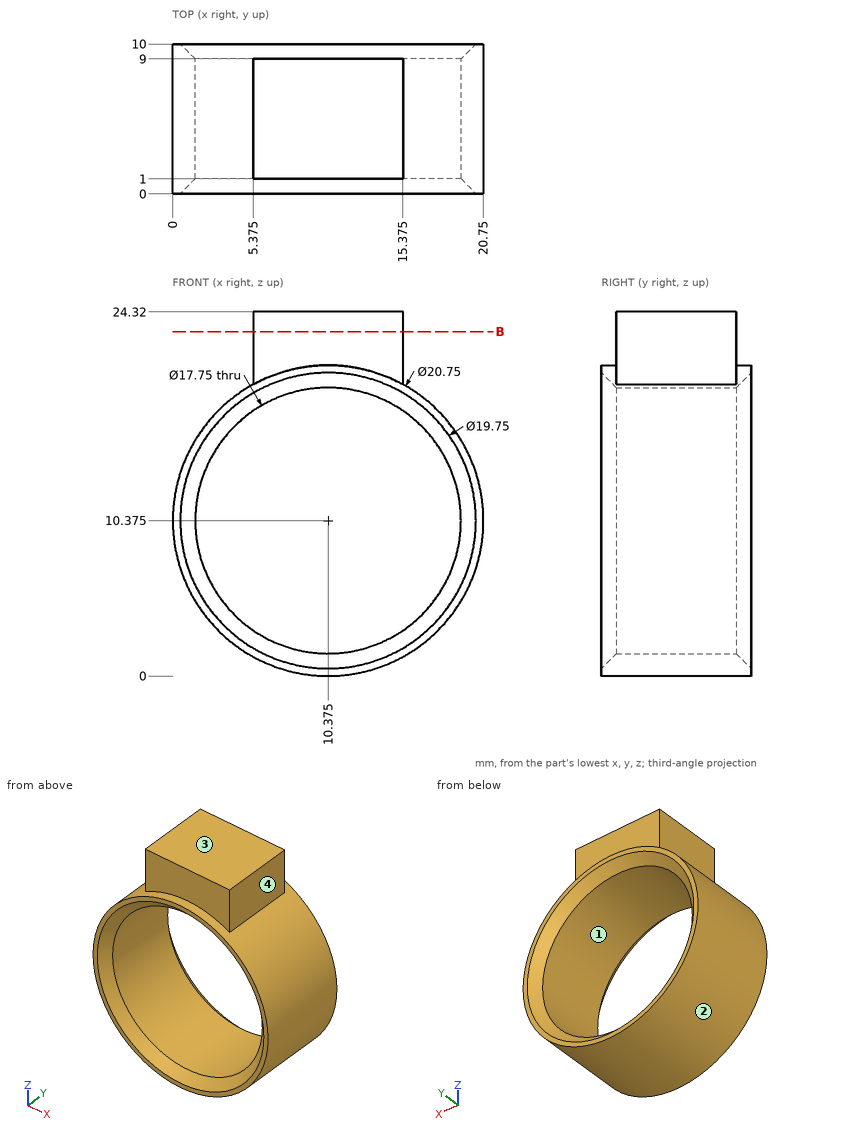
Study the drawing (mm; zero at the part's minimum x, y, z) and answer. Give positions to 0.01 mm unless a question says otherwise; leave off trailing zeros. Order: outer loops, then holes, each group sorted by start corner. A loop starts at its lowest first (then second) coordinate and runs counter-clockwise, first axis right, second up.
1) Consider line 1 along X through (y, z) = (1.5, 16.25) (1 decimal); line 2 along Z through (x, y) = (6.25, 0.5) (1 decimal); line 3 along X through (y, z) = (4.5, 17). Determine where each line is inside the solid, lowest interval first.
Reported:
line 1: x = 1.8 to 3.7, 17 to 18.9
line 2: z = 0.9 to 2, 18.8 to 19.9
line 3: x = 2.39 to 4.47, 16.28 to 18.36
2) Given P1, Ø2, axis at y = 6.5, z = 5.5, coming from the +X side; P2, Ø10, axis at x = 18, z = 16, coming from the +Y side; P3, Ø2.5, axis at y = 5.5, z = 21.5, coming from the -X side (3 decimals); P4, Ø4, axis at y = 3.5, z = 21.5, coming from the +X side (3 decimals), each flat-ended and moving along its own axis, determine where each tip first touches the part or whether it passes through.
Reported:
P1: stops at x = 20
P2: stops at y = 10
P3: stops at x = 5.375
P4: stops at x = 15.375
3) Find section B-B on z = 23. Write down the section's boundary in (x, y) (1 decimal), then the cut area to 3 significant figures.
Reported:
outline: (5.4, 1) - (15.4, 1) - (15.4, 9) - (5.4, 9) - close
area: 80.0 mm2
4) Determine the mould class of the marked faces 1, 2, 3 and 4 for opening direction Z: pulls with the +Z half, pulls with the -Z half, needs draft (parallel to the pull), parting line crosses it, or undercut.
Reported:
face 1: undercut
face 2: parting line crosses it
face 3: pulls with the +Z half
face 4: needs draft
